```python
from build123d import *

# Parameters (mm, degrees)
F1_DEPTH = 3.81
F2_R     = 1.90499
F3_R     = 3.81
F4_DEPTH = 2.54


# Not quite as in the source:
# - a fillet or chamfer is up to 0.001 mm smaller than in the source, because OpenCascade refuses the exact size
# - ends of sketch curves that miss each other by under 0.0002 mm in the source are joined


with BuildPart() as f1:
    # F0 (on Top) → F1 (new body)
    with BuildSketch(Plane.XY):
        Polygon((19.939, 0), (0, 0), (0, -3.81), (23.749, -3.81), (23.749, 6.985), (31.369, 6.985), (31.369, -14.605), (42.799, -14.605), (42.799, -10.795), (35.179, -10.795), (35.179, 10.795), (19.939, 10.795), align=None)
    extrude(amount=F1_DEPTH)

    # F2 (radius 1.905 in the source; OpenCascade refuses exactly that, so slightly less here)
    f2_edges = [f1.edges().sort_by_distance(p)[0] for p in [
        (9.9695, 0, 3.81),
        (9.9695, 0, 0),
        (11.8745, -3.81, 3.81),
        (11.8745, -3.81, 0),
        (27.559, 10.795, 3.81),
        (27.559, 6.985, 3.81),
        (27.559, 6.985, 0),
        (27.559, 10.795, 0),
        (38.989, -10.795, 3.81),
        (37.084, -14.605, 3.81),
        (38.989, -10.795, 0),
        (37.084, -14.605, 0),
    ]]
    fillet(f2_edges, radius=F2_R)

    # F3 (on face) → F4 (join)
    with BuildSketch(Plane.YZ.offset(42.799)):
        with Locations((-12.7, 1.905)):
            Circle(F3_R)
        with BuildLine():
            ThreePointArc((-12.70001, 0), (-14.0470413471, 0.5579586529), (-14.605, 1.90499))
            ThreePointArc((-14.605, 1.90499), (-14.0470413471, 3.2520413471), (-12.70001, 3.81))
            ThreePointArc((-12.70001, 3.81), (-11.3529586529, 3.2520413471), (-10.795, 1.90501))
            ThreePointArc((-10.795, 1.90501), (-11.3529586529, 0.5579586529), (-12.70001, 0))
        make_face(mode=Mode.SUBTRACT)
        with BuildLine():
            ThreePointArc((-12.70001, 3.81), (-14.0470413471, 3.2520413471), (-14.605, 1.90501))
            ThreePointArc((-14.605, 1.90501), (-14.0470413471, 0.5579586529), (-12.70001, 0))
            ThreePointArc((-12.70001, 0), (-11.3529586529, 0.5579586529), (-10.795, 1.90499))
            ThreePointArc((-10.795, 1.90499), (-11.3529586529, 3.2520413471), (-12.70001, 3.81))
        make_face()
    extrude(amount=F4_DEPTH)


solid = f1.part
```
Input: part model. Units: mm. Frame: model coordinates. A direction names the side the tool comes from. Coordinates: 2 decimals unless noted, no trailing zeros. Write each loop counter-clockwise with the first axis right and the second up, starting at its lowest first coordinate (ties: lowest second). Pieces come first, ordered by that corner, then holes. Notation, with made-up numbers: M 48.25,25 L 107.25,25 A15 cw 107.25,51 Z; hole C 22,56.25 d6. An arc over 180 degrees is marked long. Use one line per item in the form item = value.
Q1. Material intervals for probe 1 along X at (y, z) = (-2.75, 0.75); probe 2 along X at (y, z) = (-14.75, 1); probe 3 along X at (y, z) = (-9, 3.75), sorted ascending. Write a range as from..to.
Answer below:
probe_1 = 0..23.75, 31.37..35.18
probe_2 = 42.8..45.34
probe_3 = 31.37..35.18
Q2. Section C-C (z = 3). Return loops of the section in (x, y), plus the area to 3 significant figures.
Answer below:
outline = M 0,-3.46 L 23.75,-3.46 L 23.75,7.33 L 31.37,7.33 L 31.37,-14.26 L 42.8,-14.26 L 42.8,-16.35 L 45.34,-16.35 L 45.34,-9.05 L 42.8,-9.05 L 42.8,-11.14 L 35.18,-11.14 L 35.18,10.45 L 19.94,10.45 L 19.94,-0.35 L 0,-0.35 Z
area = 275 mm²
Q3. First-contact query: pin 1 (4 mm diameter, centred on y = 1, z = 1.5, fed in from +X); pin 2 (4 mm diameter, centred on y = -0.5, z = 2.5, fed in from -X); pin 3 (12 mm diameter, centred on x = 30.5, y = -1.5, fed in from -Z); pin 4 (1.9 mm diameter, centred on y = 2.5, z = 2, fed in from -X). Flat tips, straight axial feed; report the tip coordinate or a pass-through.
Answer below:
pin_1 = 35.18
pin_2 = 0
pin_3 = 0
pin_4 = 19.94
Q4. Draft query along X for faces 1 (the face through (42.799, -12, 4)), 2 (the face through (45.339, -13, 2)), 3 (the face through (38.94, -11.34, 0.57)), 4 (the face through (9.83, -0.543, 3.237)). Return one class per face: released by +X, released by -X, zero draft, split by the parting line, or undercut.
Answer below:
face_1 = undercut
face_2 = released by +X
face_3 = undercut
face_4 = zero draft
Q5. Section D-D (y = -7.75). Return loops of the section in (x, z).
Answer below:
outline = M 31.37,0 L 35.18,0 L 35.18,3.81 L 31.37,3.81 Z
Q6. Set-up query: faces 5 (the face through (27.6, 7.5, 0.6)), 6 (the face through (37.16, -14.06, 0.57)), 7 (the face through (37.16, -14.06, 3.24)), 8 (the face through (38.94, -11.34, 3.24)), 9 (the face through (44.051, -16.506, 2.073)). Return all of +Z, -Z, +X, -X, +Y, -Y with unobstructed straight access to the full face (end or side cutting, diameter ignored); none if empty.
Answer below:
face_5 = -Z, -Y
face_6 = -Z, -X, -Y
face_7 = +Z, -X, -Y
face_8 = +Z, +Y
face_9 = +X
Q7. Section B-B (y = -3). Return loops of the section in (x, z).
Answer below:
outline = M 0,0.35 L 23.75,0.35 L 23.75,3.46 L 0,3.46 Z; M 31.37,0 L 35.18,0 L 35.18,3.81 L 31.37,3.81 Z
